Verification items for this drawing (mm, ordinates from the low corner). A direction names the side the tool comes from. Round coordinates to 2 decimals unless told otherwise and drop trailing zeros. Loops run counter-clockwise (first coordinate to the right, second up) from the corner with the lowest first, then second, coordinate; pieces in that order, holes last. Notation, with made-up numbers: (-30, 9.25) - (-18, 9.25) arc R21 cw to (-18, 48.25) - close; hole circle Ø7 at (18.5, 45). An arc over 180 degrees is marked (long way). Answer in a Markdown table with one row per item. Add a question column.
(1) Gauge pin test, flat ends, axial feed: pin 1 (8 mm diameter, centred on y = 13.5, z = 15, fed in from -X); pin 2 (5 mm diameter, centred on x = 9.5, z = 11, fed in from -Y) (1 decimal). Record the tip position at first contact, or that the pin passes through.
(2) Access from +Z, -Z, +X, -X, +Y, -Y to the whole of each face (thin tool, end or side, straight path). Record for the marked faces 5 and 6.
(3) Cross-section at C-C on x = 8.5. Enter the section's corners in (y, z) (1 decimal).
(4) Thickness scan on line 1 along Y through (x, z) = (16.5, 10.75) (1 decimal); line 2 along Y through (x, z) = (2.25, 17) (1 decimal). Record the ranges inside material, lowest first.
(5) Mould release check, pull along Z, two halves, no side actions. Record for the marked faces 1, 2, 3 and 4: +Z half, -Z half, draft (parallel to the pull), parting line (faces both ways), or undercut.
(6) Cross-section at B-B on z = 8.75. Count the separate pieces of the cut face and the enclosed holes in it.
(7) Cross-section at D-D on x = 1.75. Enter the section's corners in (y, z) (1 decimal).
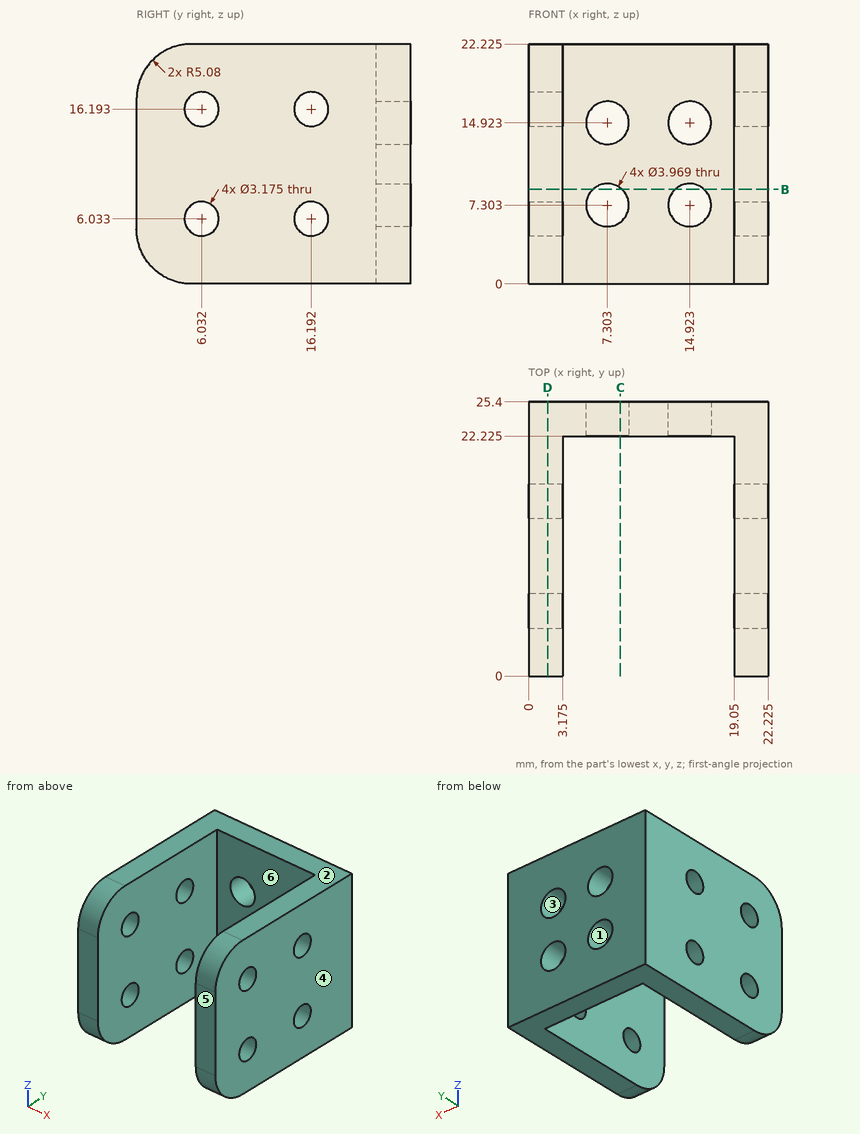
Answers:
| question | item | result |
|---|---|---|
| 1 | pin 1 | stops at x = 0 |
| 1 | pin 2 | stops at y = 22.2 |
| 2 | face 5 | +Z, -Z, +X, -X, -Y |
| 2 | face 6 | +Z, -Z, -Y |
| 3 | outline | (22.2, 0) - (25.4, 0) - (25.4, 5.7) - (22.2, 5.7) - close; (22.2, 8.9) - (25.4, 8.9) - (25.4, 13.3) - (22.2, 13.3) - close; (22.2, 16.5) - (25.4, 16.5) - (25.4, 22.2) - (22.2, 22.2) - close |
| 4 | line 1 | y = 22.2 to 25.4 |
| 4 | line 2 | y = 0 to 4.7, 7.4 to 14.8, 17.6 to 25.4 |
| 5 | face 1 | undercut |
| 5 | face 2 | +Z half |
| 5 | face 3 | undercut |
| 5 | face 4 | draft |
| 6 | separate pieces | 3 |
| 6 | enclosed holes | 0 |
| 7 | outline | (0, 5.1) arc R5.1 ccw to (5.1, 0) - (25.4, 0) - (25.4, 22.2) - (5.1, 22.2) arc R5.1 ccw to (0, 17.1) - close; hole circle Ø3.2 at (6, 6); hole circle Ø3.2 at (6, 16.2); hole circle Ø3.2 at (16.2, 6); hole circle Ø3.2 at (16.2, 16.2) |
